Build history of the part. All positions in model axes, mm. A direction names the side the tool comes from. Round coordinates to 2 decimals unless told otherwise and drop trailing zeros. Write each loop counter-clockwise with the first axis right and the second up, starting at its lowest first coordinate (ties: lowest second). Pieces come first, ordered by that corner, then holes. Notation, with made-up numbers: (-9.75, 86.25) - (-4.75, 86.25) arc R31 ccw to (-4.75, 125.25) - close; hole circle Ø5 at (20, 81.5). An arc over 180 degrees is marked (long way). One line per question, with ' | ' between items.
Autodesk Inventor part; units mm, degrees
ref_plane "YZ Plane" through (0, 0, 0) normal (1, 0, 0) x (0, 1, 0)
ref_plane "XZ Plane" through (0, 0, 0) normal (0, 1, 0) x (-1, 0, 0)
ref_plane "XY Plane" through (0, 0, 0) normal (0, 0, 1) x (1, 0, 0)
sketch "Skizze3" plane through (0, 0, 0) normal (1, 0, 0) x (0, 1, 0)
  line L0 (0, 60) -> (0, -10) construction
  line L1 (-35, 0) -> (35, 0) construction
  line L2 (25, 0) -> (25, 22.5) construction
  line L3 (25, 50) -> (-25, 50)
  line L4 (-25, 50) -> (-25, 26)
  line L5 (11.1, 0) -> (11.1, 26) construction
  line L6 (11.1, 26) -> (-11.1, 26) construction
  line L7 (-11.1, 26) -> (-11.1, 0) construction
  line L8 (11.1, 22.5) -> (25, 22.5)
  line L9 (11.1, 22.5) -> (11.1, 26)
  line L10 (11.1, 26) -> (-25, 26)
  line L11 (-25, 26) -> (-25, 0) construction
  line L12 (25, 22.5) -> (25, 50)
  point P0 (0, 0)
  dimension "d8" = 100
  dimension "d9" = 50
  dimension "d10" = 52
  dimension "d11" = 22.2
  dimension "d13" = 45
revolve "Grundkörper" add sketch "Skizze3" angle 360 about axis through (0, 0, 0) along (0, 1, 0)
sketch "Skizze4" plane through (0, 0, 0) normal (1, 0, 0) x (0, 1, 0)
  line L0 (-25, 50) -> (25, 50) construction
  line L1 (0, 48) -> (0, -8) construction
  line L2 (-15, 50) -> (-15, 30)
  line L3 (-15, 30) -> (15, 30)
  line L4 (15, 30) -> (15, 50)
  line L5 (-15, 50) -> (15, 50)
  point P0 (0, 0)
  dimension "d17" = 30
  dimension "d18" = 20
extrude "Profil_Ausschnitt" cut sketch "Skizze4" along normal through all both and the other way through all
sketch "Skizze5" plane through (0, -25, 0) normal (0, -1, 0) x (1, 0, 0)
  circle A0 centre (0, 0) radius 50 construction
  line L0 (0, 70) -> (0, -70) construction
  line L1 (-40, 30) -> (40, 30) construction
  line L2 (0, 30) -> (0, 50) construction
  point P0 (0, 40)
hole "ISO4762_M8_Boh" at (0, -25, 40) direction (0, 1, 0) diameter 9 end up to surface counterbore diameter 15 counterbore depth 5.6
mirror "Spiegelung_ISO4762_M8_Boh" about plane through (0, 0, 0) normal (0, 1, 0) of "ISO4762_M8_Boh"
sketch "Skizze7" plane through (0, 0, 0) normal (1, 0, 0) x (0, 1, 0)
  line L0 (-35, 0) -> (35, 0) construction
  line L1 (11.1, -26) -> (11.1, 26) construction
  line L2 (11.1, 26) -> (-25, 26) construction
  line L3 (-11.1, 26) -> (-11.1, 27.5)
  line L4 (-11.1, 27.5) -> (-13.25, 27.5)
  line L5 (-13.25, 27.5) -> (-13.25, 26)
  line L6 (-11.1, 26) -> (-13.25, 26)
  point P0 (0, 0)
  dimension "d34" = 55
  dimension "d35" = 2.15
  dimension "d36" = 22.2
revolve "DIN472-52x2-Nut" cut sketch "Skizze7" angle 360 about axis through (0, 0, 0) along (0, 1, 0)
chamfer "Fase_Allgemein" distance 2 angle 45 4 edges at (0, -25, -50) (0, 25, -50) (0, -25, -26) (0, 25, -22.5)
chamfer "Fase2" distance 0.2 angle 45 1 edges at (0, 11.1, -22.5)
properties part number "200-30-ROCKER-BOGIE-BEARING-01" material "Aluminium 6061"
Q1. Saw through at C-C, the plane x = 0. State how many separate pieces and enclosed holes the cut face has, then the cut area to 3 significant figures.
Found:
separate pieces: 4 | enclosed holes: 0 | area: 1,630 mm^2
Q2. Which spindle directions (+Z, -Z, +X, -X, +Y, -Y) get a long thin tool onto all of the face, cutting with end or side? Do faces 5 (the cylindrical face through (15.821, -0.155, -20.633)), 6 (the flat face through (-24.3, -11.1, 10.1)), 7 (the flat face through (5, 19.4, 40)). Say none if no direction does.
Found:
face 5: -Y | face 6: none | face 7: +Y
Q3. Pull direction Y, two halves, no side cores. Call faces 1 (the conical face through (-22.087, 23.125, -4.905)), 2 (the flat face through (-1, 0, 30)), 3 (the cylindrical face through (26.846, -12.19, -5.961)), 4 (the flat face through (-21, -25, 21)): +Y half, -Y half, draft (parallel to the pull), parting line (faces both ways), or undercut.
Found:
face 1: +Y half | face 2: undercut | face 3: undercut | face 4: -Y half
Q4. Drop flat-ended pins along their axis: pin 1 (8 mm diameter, centred on x = 27, y = -1, fed in from +Z); pin 2 (12 mm diameter, centred on y = 19.5, z = 39, fed in from +X); pin 3 (7.5 mm diameter, centred on x = 0, z = 42, fed in from +Y); pin 4 (8 mm diameter, centred on x = 0, z = 40, fed in from +Y). Give the stop position or say it passes through.
Found:
pin 1: z = 30 | pin 2: x = 37.56 | pin 3: y = 19.4 | pin 4: through
Q5. Drill centre lines: L1, parallel to Z at x = 5.5, y = 22.5; L2, parallel to X at y = -20, z = 0; L3, parallel to Y at x = -5.5, z = 40. Where is each one in solid material? Low to high. Write a range as from..to.
Found:
L1: -49.7..-21.82, 21.82..34.9, 45.1..49.7 | L2: -50..-26, 26..50 | L3: -19.4..-15, 15..19.4
Q6. Saw through at B-B, the plane y = -6. List the corners of the cut face in (x, z), then the cut area to 3 significant figures.
Found:
outline: (-40, 30) arc R50 ccw (long way) to (40, 30) - close; hole circle Ø52 at (0, 0) | area: 4,610 mm^2
